CAD build for the part. Positions are in the model's coordinates, mm. Face numbers are marked on the shaded views. Round coordinates to 2 decimals unless told otherwise and drop trailing zeros. Write each question's results on one line, items separated by ' | '. Start each with the question number.
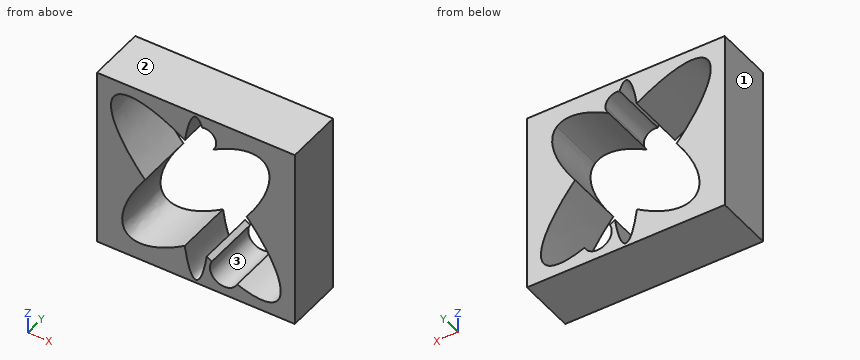
```python
from build123d import *

# Parameters (mm, degrees)
F0_W     = 86.713158
F0_H     = 79.58214
F1_DEPTH = 25.4


with BuildPart() as f1:
    # F0 (on Front) → F1 (new body)
    with BuildSketch(Plane.XZ):
        Rectangle(F0_W, F0_H)
        with BuildLine():
            add(Edge.make_bspline(
                [(-35.36984, 32.660052), (-43.630681, 23.713813), (-22.259437, -1.337829)],
                knots=[0, 0, 0, 1.244177, 1.244177, 1.244177], degree=2, weights=[1, 0.812663, 1]))
            add(Edge.make_bspline(
                [(-4.765757, 25.279926), (-28.087234, 40.546892), (-35.36984, 32.660052)],
                knots=[5.155733, 5.155733, 5.155733, 6.283185, 6.283185, 6.283185], degree=2, weights=[1, 0.84527, 1]))
            add(Edge.make_bspline(
                [(0, 38.364865), (-2.872782, 38.364865), (-4.765757, 25.279926)],
                knots=[0, 0, 0, 0.851395, 0.851395, 0.851395], degree=2, weights=[1, 0.910751, 1]))
            add(Edge.make_bspline(
                [(2.763368, 34.523458), (1.454502, 38.364865), (0, 38.364865)],
                knots=[5.831864, 5.831864, 5.831864, 6.283185, 6.283185, 6.283185], degree=2, weights=[1, 0.974647, 1]))
            ThreePointArc((2.763368, 34.523458), (7.020907, 33.649159), (8.935218, 29.747051))
            ThreePointArc((8.935218, 29.747051), (8.539057, 27.809914), (7.41419, 26.183841))
            add(Edge.make_bspline(
                [(30.235512, 30.092888), (24.193663, 36.163372), (7.41419, 26.183841)],
                knots=[0, 0, 0, 0.981014, 0.981014, 0.981014], degree=2, weights=[1, 0.882094, 1]))
            add(Edge.make_bspline(
                [(22.259437, 1.337829), (37.712849, 22.580113), (30.235512, 30.092888)],
                knots=[5.115155, 5.115155, 5.115155, 6.283185, 6.283185, 6.283185], degree=2, weights=[1, 0.834256, 1]))
            add(Edge.make_bspline(
                [(18.116728, -32.437346), (68.240774, -52.562076), (22.259437, 1.337829)],
                knots=[2.394352, 2.394352, 2.394352, 4.38577, 4.38577, 4.38577], degree=2, weights=[1, 0.543908, 1]))
            ThreePointArc((18.116728, -32.437346), (9.559764, -35.369126), (6.991325, -26.696173))
            add(Edge.make_bspline(
                [(4.765757, -25.279926), (5.883942, -26.011924), (6.991325, -26.696173)],
                knots=[2.01414, 2.01414, 2.01414, 2.074741, 2.074741, 2.074741], degree=2, weights=[1, 0.999541, 1]))
            add(Edge.make_bspline(
                [(-4.862435, -24.595616), (-0.11439, -59.013299), (4.765757, -25.279926)],
                knots=[2.266724, 2.266724, 2.266724, 3.992988, 3.992988, 3.992988], degree=2, weights=[1, 0.650061, 1]))
            add(Edge.make_bspline(
                [(-22.259437, -1.337829), (-69.92987, -66.86568), (-4.862435, -24.595616)],
                knots=[1.973562, 1.973562, 1.973562, 4.203143, 4.203143, 4.203143], degree=2, weights=[1, 0.440366, 1]))
        make_face(mode=Mode.SUBTRACT)
    extrude(amount=F1_DEPTH)


solid = f1.part
```
1) Saw through at A-A, the plane z = -28. State how many separate pieces and enclosed holes the cut face has, plus the area to 3 significant figures.
2) Wall check: line 1 along Z through (x, y) = (-27.5, -6); line 2 along X through (y, z) = (-12, 27); line 3 along X through (y, z) = (-23, 8). Give the ranges that are in metal, low to high. Write a range as from..to.
3) Pull direction Z, two halves, no side cores. Call the marked faces 1, 2 and 3: pulls with the +Z half, pulls with the -Z half, needs draft (parallel to the pull), parting line crosses it, or undercut.
Filled sheet:
1) separate pieces: 4 | enclosed holes: 0 | area: 670 mm^2
2) line 1: z = -39.79..-31.72, -9.52..5.3, 34.9..39.79 | line 2: x = -43.36..-37.2, -7.49..-4.5, 8.1..8.82, 31.95..43.36 | line 3: x = -43.36..-29.38, 26.64..43.36
3) face 1: needs draft | face 2: pulls with the +Z half | face 3: undercut
